Geometry: see drawing. Coordinates: mm, zero at the bounding-box minimum. Round coordinates to 2 decimals unless told otherwise and drop trailing zeros. Order: outer loops, then holes, each group sorted by start corner. A loop starts at its lowest first (then second) coordinate and runs counter-clockwise, first axis right, second up. Notation, with made-up numbers: (22, 77.25) -> (37, 77.25) arc R27 cw to (37, 110.25) -> close; hole circle Ø5 at (4.25, -5.5). An arc over 180 degrees is marked (long way). Use a Markdown table: item, result.
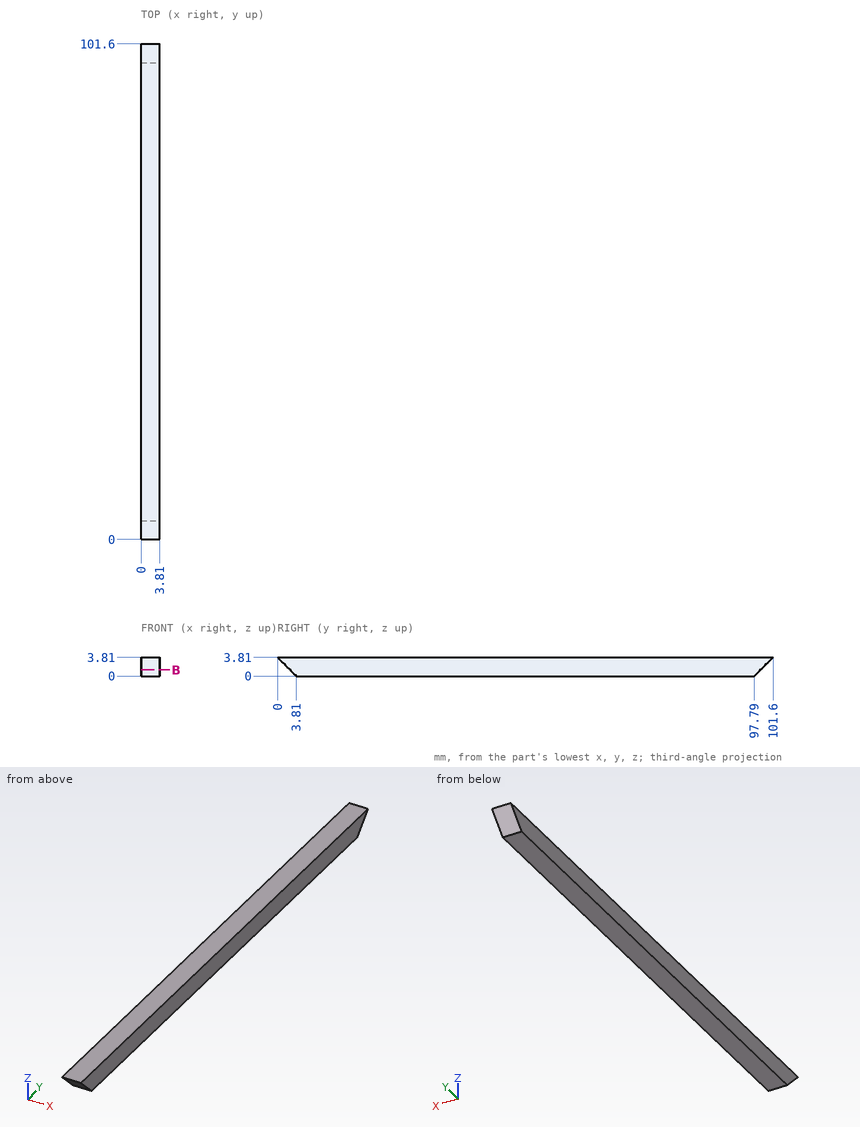
1) Ray query, probe 1 along Y at (x, z) = (1.85, 3.55); probe 2 along Y at (x, z) = (1.95, 1.4). Return the intervals inside material, ascending.
Answer key:
| item | result |
|---|---|
| probe 1 | y = 0.26 to 101.34 |
| probe 2 | y = 2.41 to 99.19 |
2) Contact query for flat-ended pins moving along their axis: P1, Ø1, axis at x = 2, z = 3, coming from the -Y side; P2, Ø1, axis at x = 0.5, z = 3, coming from the +Y side. Output: stop coordinate, or through.
Answer key:
| item | result |
|---|---|
| P1 | stops at y = 0.31 |
| P2 | stops at y = 101.29 |
3) Cut plane B-B on z = 1.25. Return loops of the section in (x, y).
Answer key:
| item | result |
|---|---|
| outline | (0, 2.56) -> (3.81, 2.56) -> (3.81, 99.04) -> (0, 99.04) -> close |
